```python
from build123d import *

# Parameters (mm, degrees)
SKETCH1_W           = 229
SKETCH1_H           = 25
BOSS_EXTRUDE1_DEPTH = 23
CUT_EXTRUDE1_DEPTH  = 23


with BuildPart() as part:
    # Sketch1 → Boss-Extrude1 (new body)
    with BuildSketch(Plane.XY):
        with Locations((114.5, 12.5)):
            Rectangle(SKETCH1_W, SKETCH1_H)
    extrude(amount=BOSS_EXTRUDE1_DEPTH)

    # Sketch2 → Cut-Extrude1 (cut)
    with BuildSketch(Plane.XY.offset(23)):
        Polygon((43.428571429, 21.197944284), (35.928571429, 16.867817265), (35.928571429, 8.207563227), (43.428571429, 3.877436208), (50.928571429, 8.207563227), (50.928571429, 16.867817265), align=None)
        Polygon((15, 3.839745962), (22.5, 8.169872981), (22.5, 16.830127019), (15, 21.160254038), (7.5, 16.830127019), (7.5, 8.169872981), align=None)
        Polygon((71.857142857, 21.235634529), (64.357142857, 16.90550751), (64.357142857, 8.245253472), (71.857142857, 3.915126454), (79.357142857, 8.245253472), (79.357142857, 16.90550751), align=None)
        Polygon((100.285714286, 21.273324775), (92.785714286, 16.943197756), (92.785714286, 8.282943718), (100.285714286, 3.952816699), (107.785714286, 8.282943718), (107.785714286, 16.943197756), align=None)
        Polygon((128.714285714, 21.311015021), (121.214285714, 16.980888002), (121.214285714, 8.320633964), (128.714285714, 3.990506945), (136.214285714, 8.320633964), (136.214285714, 16.980888002), align=None)
        Polygon((157.142857143, 21.348705266), (149.642857143, 17.018578247), (149.642857143, 8.358324209), (157.142857143, 4.028197191), (164.642857143, 8.358324209), (164.642857143, 17.018578247), align=None)
        Polygon((185.571428571, 21.386395512), (178.071428571, 17.056268493), (178.071428571, 8.396014455), (185.571428571, 4.065887436), (193.071428571, 8.396014455), (193.071428571, 17.056268493), align=None)
        Polygon((214, 21.424085758), (206.5, 17.093958739), (206.5, 8.433704701), (214, 4.103577682), (221.5, 8.433704701), (221.5, 17.093958739), align=None)
    extrude(amount=-CUT_EXTRUDE1_DEPTH, mode=Mode.SUBTRACT)


solid = part.part
```
Design review of the part built by this model. Coordinates are the model's own, in mm. A direction names the side the tool comes from. Coordinates: 2 decimals unless noted, no trailing zeros. Loops run counter-clockwise (first coordinate to the right, second up) from the corner with the lowest first, then second, coordinate; pieces in that order, holes last.
Q1. Tool access review of faces 4 (the face through (113, 25, 11)), 5 (the face through (104.088, 19.078, 11.661)): name each direction out of +Z, -Z, +X, -X, +Y, -Y from which nothing blocks a thin tool from reaching the whole face with its end or side.
Reported:
face 4: +Z, -Z, +X, -X, +Y
face 5: +Z, -Z
Q2. We need section B-B on x = 134. State the section outline as (y, z) points, and give its area (3 significant figures).
Reported:
outline: (0, 0) - (7.04, 0) - (7.04, 23) - (0, 23) - close; (18.26, 0) - (25, 0) - (25, 23) - (18.26, 23) - close
area: 317 mm2
Q3. We need section A-A on y = 13. State how many separate pieces and enclosed holes the cut face has, and give its area (3 significant figures).
Reported:
separate pieces: 9
enclosed holes: 0
area: 2,510 mm2
Q4. To check wall thickness, follow line 1 (Y direction, x = 160, z = 5.5); line 2 (Y direction, x = 73, z = 3.5). State the ranges of each line that lie inside material, in increasing order.
Reported:
line 1: y = 0 to 5.68, 19.7 to 25
line 2: y = 0 to 4.57, 20.58 to 25
Q5. The part is to be moulded in two halves that separate along X. For faces 1 (the face through (113, 0, 11)), 2 (the face through (0, 12, 11)), 3 (the face through (64.357, 13, 12)), say which applies: +X half, -X half, draft (parallel to the pull), parting line (faces both ways), or undercut.
Reported:
face 1: draft
face 2: -X half
face 3: undercut
